Model file for the job. Use its own axes, mm. A direction names the side the tool comes from. Coordinates: 2 decimals unless noted, no trailing zeros. Write each loop counter-clockwise with the first axis right and the second up, starting at its lowest first coordinate (ties: lowest second). Pieces come first, ordered by that corner, then holes. Notation, with made-up numbers: M 31,71.5 L 68,71.5 A21 ccw 68,88.5 Z; hole C 13.25,-3.75 d4. An arc over 180 degrees is marked long. Answer in a Markdown table with one row per item. Add a question column.
```python
from build123d import *

# Parameters (mm, degrees)
SKETCH_1_W          = 200
SKETCH_1_H          = 200
EXTRUDE_1_DEPTH     = 10
SKETCH_2_W          = 10.2
SKETCH_2_H          = 10.2
CUT_EXTRUDE_3_DEPTH = 5
FILLET_1_R          = 10
SKETCH_3_R          = 5.1
CUT_EXTRUDE_1_DEPTH = 5
SKETCH_4_R          = 2.5
CUT_EXTRUDE_2_DEPTH = 142.774468788
SKETCH_5_R          = 1.5
CUT_EXTRUDE_4_DEPTH = 142.774468788


with BuildPart() as part:
    # ｽｹｯﾁ1 → ﾎﾞｽ - 押し出し1 (new body)
    with BuildSketch(Plane(origin=(0, 0, 0), x_dir=(1, 0, 0), z_dir=(0, 1, 0))):
        Rectangle(SKETCH_1_W, SKETCH_1_H)
    extrude(amount=EXTRUDE_1_DEPTH)

    # ｽｹｯﾁ2 → ｶｯﾄ - 押し出し3 (cut)
    with BuildSketch(Plane(origin=(0, 10, 0), x_dir=(1, 0, 0), z_dir=(0, 1, 0))):
        with Locations((-85, -15)):
            Rectangle(SKETCH_2_W, SKETCH_2_H)
        with Locations((85, -15)):
            Rectangle(SKETCH_2_W, SKETCH_2_H)
        with Locations((-85, -85)):
            Rectangle(SKETCH_2_W, SKETCH_2_H)
        with Locations((85, -85)):
            Rectangle(SKETCH_2_W, SKETCH_2_H)
    extrude(amount=-CUT_EXTRUDE_3_DEPTH, mode=Mode.SUBTRACT)

    # ﾌｨﾚｯﾄ1
    fillet_1_edges = [part.edges().sort_by_distance(p)[0] for p in [
        (100, 5, 100),
        (-100, 5, 100),
        (-100, 5, -100),
        (100, 5, -100),
    ]]
    fillet(fillet_1_edges, radius=FILLET_1_R)

    # ｽｹｯﾁ3 → ｶｯﾄ - 押し出し1 (cut)
    with BuildSketch(Plane(origin=(0, 10, 0), x_dir=(1, 0, 0), z_dir=(0, 1, 0))):
        with Locations(Location((-85, 85, 0), (0, 0, 270))):
            Circle(SKETCH_3_R)
        with Locations(Location((85, 85, 0), (0, 0, 270))):
            Circle(SKETCH_3_R)
        with Locations(Location((-85, 15, 0), (0, 0, 270))):
            Circle(SKETCH_3_R)
        with Locations(Location((85, 15, 0), (0, 0, 270))):
            Circle(SKETCH_3_R)
    extrude(amount=-CUT_EXTRUDE_1_DEPTH, mode=Mode.SUBTRACT)

    # ｽｹｯﾁ4 → ｶｯﾄ - 押し出し2 (cut, through all)
    with BuildSketch(Plane(origin=(0, 10, 0), x_dir=(1, 0, 0), z_dir=(0, 1, 0))):
        with Locations(Location((-68, -38, 0), (0, 0, 270))):
            Circle(SKETCH_4_R)
        with Locations(Location((-68, -62, 0), (0, 0, 270))):
            Circle(SKETCH_4_R)
        with Locations(Location((-92, -62, 0), (0, 0, 270))):
            Circle(SKETCH_4_R)
        with Locations(Location((-92, -38, 0), (0, 0, 270))):
            Circle(SKETCH_4_R)
    extrude(amount=-CUT_EXTRUDE_2_DEPTH, mode=Mode.SUBTRACT)

    # ｽｹｯﾁ5 → ｶｯﾄ - 押し出し4 (cut, through all)
    with BuildSketch(Plane.XZ):
        with Locations(Location((-85, 85, 0), (0, 0, 270))):
            Circle(SKETCH_5_R)
        with Locations(Location((85, 85, 0), (0, 0, 270))):
            Circle(SKETCH_5_R)
        with Locations(Location((-85, 15, 0), (0, 0, 270))):
            Circle(SKETCH_5_R)
        with Locations(Location((85, 15, 0), (0, 0, 270))):
            Circle(SKETCH_5_R)
    extrude(amount=-CUT_EXTRUDE_4_DEPTH, mode=Mode.SUBTRACT)


solid = part.part
```
1) Two-plate mould, pull along X, no slides. Class faces 3 (the face through (100, 5, 1)), 4 (the face through (-90.1, 8, 15)), 5 (the face through (-1, 5, 100)), 6 (the face through (-97.15, 5.07, 96.99)): released by +X, released by -X, zero draft, split by the parting line, or undercut.
2) Drill centre lines: probe 1 along X at (y, z) = (1.6, 15); probe 2 along X at (y, z) = (3.5, 38); probe 3 along Z at (x, y) = (85, 3.05). Where is each one in solid material? Low to high.
3) Slice it at B-B (z = 38). Give the cut face in (x, y).
4) Slice it at A-A (x = -68). Give the cut face in (y, z), then the cut area to 3 significant figures.
5) Which spindle directions (+Z, -Z, +X, -X, +Y, -Y) get a long thin tool onto all of the face, cutting with end or side? Do faces 1 (the face through (85, 5, -15)), 2 (the face through (-1, 10, -1)). Say none if no direction does.
6) Flat gauge pin, fed straight in: pin 1 Ø3 at (x, z) = (83, 17.5) entering from +Y. Where does the tip first touch, or does it go through?
Ans:
| question | item | result |
|---|---|---|
| 1 | face 3 | released by +X |
| 1 | face 4 | undercut |
| 1 | face 5 | zero draft |
| 1 | face 6 | released by -X |
| 2 | probe 1 | x = -100 to -86.5, -83.5 to 83.5, 86.5 to 100 |
| 2 | probe 2 | x = -100 to -94.5, -89.5 to -70.5, -65.5 to 100 |
| 2 | probe 3 | z = -100 to 13.5, 16.5 to 83.5, 86.5 to 100 |
| 3 | outline | M -100,0 L -94.5,0 L -94.5,10 L -100,10 Z; M -89.5,0 L -70.5,0 L -70.5,10 L -89.5,10 Z; M -65.5,0 L 100,0 L 100,10 L -65.5,10 Z |
| 4 | outline | M 0,-100 L 10,-100 L 10,35.5 L 0,35.5 Z; M 0,40.5 L 10,40.5 L 10,59.5 L 0,59.5 Z; M 0,64.5 L 10,64.5 L 10,100 L 0,100 Z |
| 4 | area | 1,900 mm2 |
| 5 | face 1 | +Y |
| 5 | face 2 | +Z, -Z, +X, -X, +Y |
| 6 | pin 1 | stops at y = 5 |
